Read the model definition and answer for the solid it produces. Units are mm, in the model's axes. Face numbers are marked on the shaded views. A direction names the side the tool comes from. Round coordinates to 2 decimals unless told otherwise and drop trailing zeros. Write each loop counter-clockwise with the first axis right and the second up, starting at its lowest first coordinate (ties: lowest second). Pieces come first, ordered by that corner, then holes. Notation, with made-up numbers: (72, 7) - (99, 7) arc R28 ccw to (99, 43) - close; hole circle Ø5 at (6.5, -25). An arc over 180 degrees is marked (long way). One line per item, written item: value. Start each with the question number.
(1) Flat-ended cylindrical pins translate along their axes: pin 1 Ø0.6 at (x, y) = (0, -0.5) entering from -Z; pin 2 Ø1.5 at (x, z) = (1, -6.5) entering from +Y; pin 3 Ø1 at (y, z) = (1, -4) entering from -X. Find the tip coordinate at first contact, or state that the pin passes through.
(2) A cutting plane is placed at D-D, the plane x = -1.2. Determine the outline of the cut face in (y, z).
(3) A cutting plane is placed at C-C, the plane y = 0. Determine the outline of the cut face in (x, z), plus the area to 3 significant figures.
(4) Find the intervals of material crossed by L1, parallel to Z at x = 0, y = 1.3; L2, parallel to Z at x = 0.65, y = 0.8; L3, parallel to Y at x = 0, z = -3.5, in increasing order.
(5) A cutting plane is placed at A-A, the plane z = -0.75. Determine the outline of the cut face in (x, y), plus the area to 3 significant figures.
(6) A cutting plane is placed at B-B, the plane y = 1.2. Determine the outline of the cut face in (x, z), plus the area to 3 significant figures.
(7) For the marked faces 1, 2 and 3, determine the directions among +Z, -Z, +X, -X, +Y, -Y from which every point of the face is accessible in a straight line to the end or side of a thin tool.
from build123d import *

# Parameters (mm, degrees)
TAGLIO_ESTRUSIONE1_DEPTH      = 9.653279386
TAGLIO_ESTRUSIONE1_DEPTH_BACK = 9.653279386
SCHIZZO2_R                    = 0.75


with BuildPart() as part:
    # Schizzo1 → Rivoluzione1 (revolve)
    with BuildSketch(Plane(origin=(0, 0, 0), x_dir=(0, 0, -1), z_dir=(1, 0, 0)), mode=Mode.PRIVATE) as rivoluzione1_sk:
        with BuildLine():
            Line((8.389233822, 1.5), (-1.610766178, 1.5))
            Line((-1.610766178, 1.5), (-1.610766178, 1))
            Line((-1.610766178, 1), (-3.610766178, 1))
            ThreePointArc((-3.610766178, 1), (-5.264033301, 1.401258538), (-6.228800167, 0))
            Line((-6.228800167, 0), (-0.610766178, 0))
            Line((-0.610766178, 0), (-0.610766178, 1))
            Line((-0.610766178, 1), (8.389233822, 1))
            Line((8.389233822, 1), (8.389233822, 1.5))
        make_face()
    revolve(rivoluzione1_sk.sketch.rotate(Axis((0, 0, 6.228800167), (0, 0, -1)), 90), axis=Axis((0, 0, 6.228800167), (0, 0, -1)))

    # Schizzo2 → Taglio-Estrusione1 (cut, two sides: drawn at the far end of the back side and taken through both)
    with BuildSketch(Plane(origin=(0, 0, 0), x_dir=(1, 0, 0), z_dir=(0, 1, 0)).offset(-TAGLIO_ESTRUSIONE1_DEPTH_BACK)):
        with Locations(Location((0, 0.139233822, 0), (0, 0, 270))):
            Circle(SCHIZZO2_R)
    extrude(amount=TAGLIO_ESTRUSIONE1_DEPTH + TAGLIO_ESTRUSIONE1_DEPTH_BACK, mode=Mode.SUBTRACT)


solid = part.part
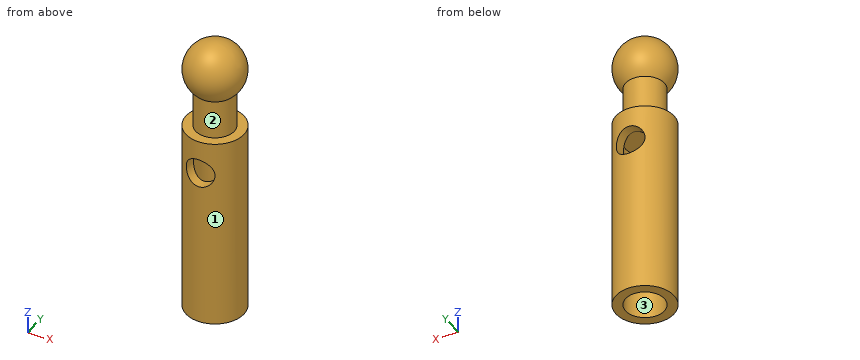
Here are the results:
1. pin 1: z = 0.61
1. pin 2: y = 1.48
1. pin 3: x = -1.41
2. outline: (-0.9, -8.39) - (0.9, -8.39) - (0.9, 1.61) - (-0.9, 1.61) - close; circle Ø1.8 at (0, 4.73)
3. outline: (-1.5, -8.39) - (-1, -8.39) - (-1, 0.61) - (1, 0.61) - (1, -8.39) - (1.5, -8.39) - (1.5, 1.61) - (1, 1.61) - (1, 3.61) arc R1.5 ccw (long way) to (-1, 3.61) - (-1, 1.61) - (-1.5, 1.61) - close
3. area: 22.5 mm²
4. L1: -8.39 to -0.89, 0.61 to 1.61, 3.98 to 5.48
4. L2: -8.39 to -0.51, 0.23 to 1.61, 3.64 to 5.82
4. L3: -1.5 to -1, 1 to 1.5
5. outline: (-0.44, -1.44) - (-0.44, -0.9) arc R1 cw to (-0.44, 0.9) - (-0.44, 1.44) arc R1.5 ccw to start; (0.44, -1.44) arc R1.5 ccw to (0.44, 1.44) - (0.44, 0.9) arc R1 cw to (0.44, -0.9) - close
5. area: 3.04 mm²
6. outline: (-0.9, -8.39) - (0.9, -8.39) - (0.9, 1.61) - (-0.9, 1.61) - close; circle Ø1.8 at (0, 4.73); hole circle Ø1.5 at (0, -0.14)
6. area: 18.8 mm²
7. face 1: +Z, -Z
7. face 2: none
7. face 3: -Z
